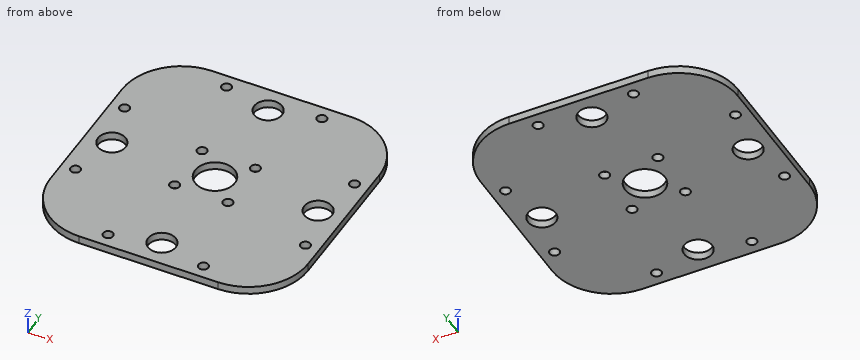
```python
from build123d import *

# Parameters (mm, degrees)
CROQUIS1_W              = 65
CROQUIS1_H              = 65
CROQUIS1_R              = 5
CROQUIS1_R_2            = 1.25
SALIENTE_EXTRUIR1_DEPTH = 2
REDONDEO1_R             = 15
CROQUIS2_R              = 3.5
CORTAR_EXTRUIR1_DEPTH   = 2
CROQUIS3_R              = 1.25
CORTAR_EXTRUIR2_DEPTH   = 2


with BuildPart() as part:
    # Croquis1 → Saliente-Extruir1 (new body)
    with BuildSketch(Plane.XY):
        Rectangle(CROQUIS1_W, CROQUIS1_H)
        Circle(CROQUIS1_R, mode=Mode.SUBTRACT)
        with Locations((-6.717514421, 6.717514421)):
            Circle(CROQUIS1_R_2, mode=Mode.SUBTRACT)
        with Locations((6.717514421, 6.717514421)):
            Circle(CROQUIS1_R_2, mode=Mode.SUBTRACT)
        with Locations((6.717514421, -6.717514421)):
            Circle(CROQUIS1_R_2, mode=Mode.SUBTRACT)
        with Locations((-6.717514421, -6.717514421)):
            Circle(CROQUIS1_R_2, mode=Mode.SUBTRACT)
    extrude(amount=SALIENTE_EXTRUIR1_DEPTH)

    # Redondeo1
    redondeo1_edges = [part.edges().sort_by_distance(p)[0] for p in [
        (32.5, -32.5, 1),
        (-32.5, -32.5, 1),
        (-32.5, 32.5, 1),
        (32.5, 32.5, 1),
    ]]
    fillet(redondeo1_edges, radius=REDONDEO1_R)

    # Croquis2 → Cortar-Extruir1 (cut)
    with BuildSketch(Plane.XY.offset(2)):
        with Locations((-26, 0)):
            Circle(CROQUIS2_R)
        with Locations((0, 26)):
            Circle(CROQUIS2_R)
        with Locations((26, 0)):
            Circle(CROQUIS2_R)
        with Locations((0, -26)):
            Circle(CROQUIS2_R)
    extrude(amount=-CORTAR_EXTRUIR1_DEPTH, mode=Mode.SUBTRACT)

    # Croquis3 → Cortar-Extruir2 (cut)
    with BuildSketch(Plane.XY.offset(2)):
        with Locations((-28.991378029, 12.02081528)):
            Circle(CROQUIS3_R)
        with Locations(Location((-12.02081528, 28.991378029, 0), (0, 0, 180))):
            Circle(CROQUIS3_R)
        with Locations((12.02081528, 28.991378029)):
            Circle(CROQUIS3_R)
        with Locations(Location((28.991378029, 12.02081528, 0), (0, 0, 180))):
            Circle(CROQUIS3_R)
        with Locations((28.991378029, -12.02081528)):
            Circle(CROQUIS3_R)
        with Locations(Location((12.02081528, -28.991378029, 0), (0, 0, 180))):
            Circle(CROQUIS3_R)
        with Locations((-12.02081528, -28.991378029)):
            Circle(CROQUIS3_R)
        with Locations(Location((-28.991378029, -12.02081528, 0), (0, 0, 180))):
            Circle(CROQUIS3_R)
    extrude(amount=-CORTAR_EXTRUIR2_DEPTH, mode=Mode.SUBTRACT)


solid = part.part
```
Source: CAD feature listing. Evaluate the final solid. Frame: model axes, mm. Round coordinates to 2 decimals unless told otherwise and drop trailing zeros. Loops run counter-clockwise (first coordinate to the right, second up) from the corner with the lowest first, then second, coordinate; pieces in that order, holes last.
1. Section query A-A on y = 0. Output: boundary loops of the cut face in (x, z).
2. Section query C-C on z = 0.9. Give the number of separate pieces and of enclosed holes in the cut face, and give its area (3 significant figures).
3. Ray query, L1, parallel to X at y = 12, z = 1.85; L2, parallel to X at y = 1, z = 1.1; L3, parallel to X at y = -28, z = 0.9. Return the intervals inside material, ascending.
4. Section query D-D on y = -23.5. Output: boundary loops of the cut face in (x, z).
Answers below:
1. outline: (-32.5, 0) - (-29.5, 0) - (-29.5, 2) - (-32.5, 2) - close; (-22.5, 0) - (-5, 0) - (-5, 2) - (-22.5, 2) - close; (5, 0) - (22.5, 0) - (22.5, 2) - (5, 2) - close; (29.5, 0) - (32.5, 0) - (32.5, 2) - (29.5, 2) - close
2. separate pieces: 1
2. enclosed holes: 17
2. area: 3,740 mm2
3. L1: x = -32.5 to -30.24, -27.74 to 27.74, 30.24 to 32.5
3. L2: x = -32.5 to -29.35, -22.65 to -4.9, 4.9 to 22.65, 29.35 to 32.5
3. L3: x = -28.21 to -12.78, -11.26 to -2.87, 2.87 to 11.26, 12.78 to 28.21
4. outline: (-31.25, 0) - (-2.45, 0) - (-2.45, 2) - (-31.25, 2) - close; (2.45, 0) - (31.25, 0) - (31.25, 2) - (2.45, 2) - close
